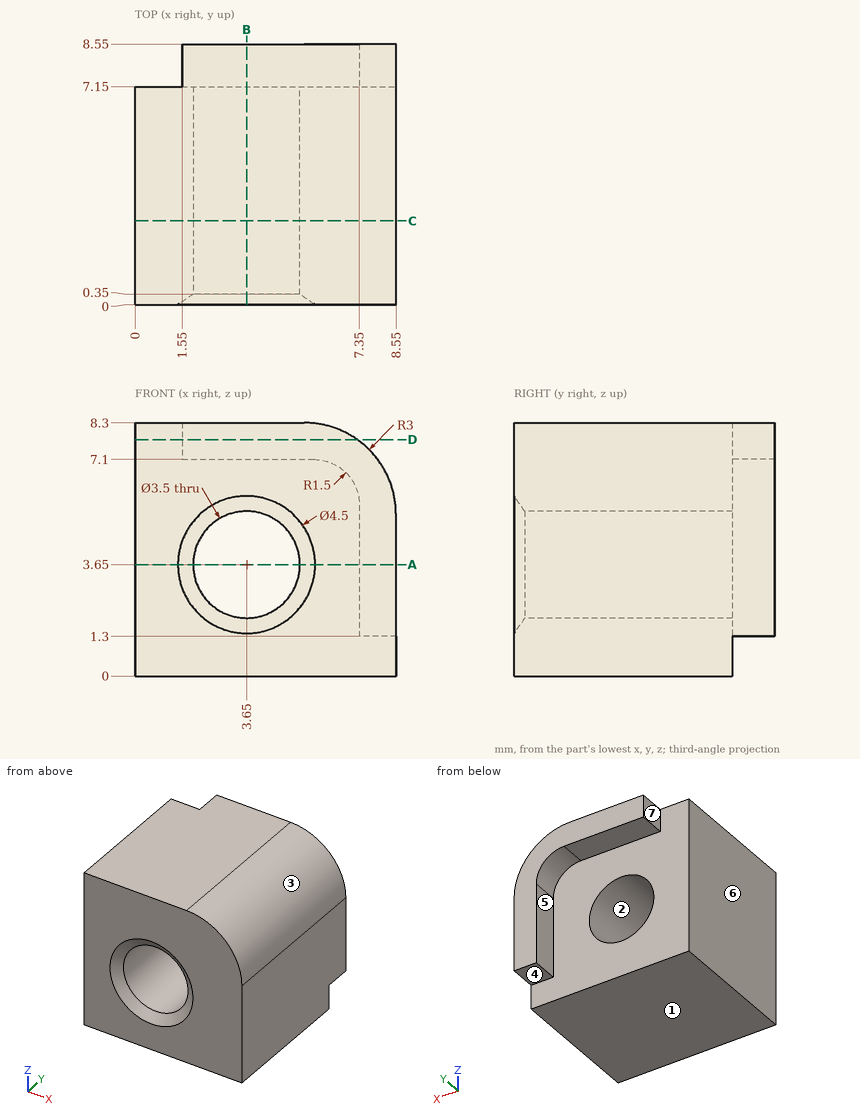
Input: dimensioned drawing with shaded views. Units: mm. Origin: part minimum x, y, z. A direction names the side the tool comes from. Give positions to 0.01 mm unless a question says otherwise; leave off trailing zeros. Order: outer loops, then holes, each group sorted by start corner. A loop starts at its lowest first (then second) coordinate and runs counter-clockwise, first axis right, second up. Notation, with made-up numbers: (68.25, -29.5) -> (85.25, -29.5) arc R20 cw to (85.25, -7.5) -> close; hole circle Ø3 at (-33, -33.5). An arc over 180 degrees is marked (long way). Use a Markdown table: item, result.
1) Ray query, line 1 along Z through (x, y) = (3.65, 3); line 2 along Y through (x, z) = (1, 0.5); line 3 along X through (y, z) = (1.5, 5.25). Return the intervals inside material, ascending. Write a range as [from, to].
Answer list:
| item | result |
|---|---|
| line 1 | [0, 1.9], [5.4, 8.3] |
| line 2 | [0, 7.15] |
| line 3 | [0, 2.94], [4.36, 8.55] |
2) Reachability of the marked faces 4, 5, 6 and 7 from +Z, -Z, +X, -X, +Y, -Y: full face, straight path, thin tool, end or side. Return the list, or none.
Answer list:
| item | result |
|---|---|
| face 4 | -Z, +X, -X, +Y |
| face 5 | -Z, -X, +Y |
| face 6 | +Z, -Z, -X, +Y, -Y |
| face 7 | +Z, -Z, -X, +Y |
3) Section query A-A, the plane z = 3.65. Return the cut outline in (x, y), then the cut area to 3 significant figures.
Answer list:
| item | result |
|---|---|
| outline | (0, 0) -> (1.4, 0) -> (1.9, 0.35) -> (1.9, 7.15) -> (0, 7.15) -> close; (5.4, 0.35) -> (5.9, 0) -> (8.55, 0) -> (8.55, 8.55) -> (7.35, 8.55) -> (7.35, 7.15) -> (5.4, 7.15) -> close |
| area | 37.6 mm² |
4) Contact query for flat-ended pins moving along their axis: P1, Ø1, axis at y = 4.5, z = 7, coming from the +X side; P2, Ø1, axis at y = 8, z = 7.5, coming from the -X side; P3, Ø1.5, axis at x = 4.5, z = 3.5, coming from the +Y side; P4, Ø1.5, axis at x = 3, y = 8, coming from the -Z side. Output: stop coordinate, or through.
Answer list:
| item | result |
|---|---|
| P1 | x = 8.3 |
| P2 | x = 1.55 |
| P3 | through |
| P4 | z = 7.1 |
5) Mould query, pull axis X, two halves, no side actions, for the marked faces 1, 2 and 3. Classes: +X half, -X half, draft (parallel to the pull), parting line (faces both ways), or undercut.
Answer list:
| item | result |
|---|---|
| face 1 | draft |
| face 2 | undercut |
| face 3 | +X half |
6) Section query C-C, the plane y = 2.75. Return the cut outline in (x, z), then the cut area to 3 significant figures.
Answer list:
| item | result |
|---|---|
| outline | (0, 0) -> (8.55, 0) -> (8.55, 5.3) arc R3 ccw to (5.55, 8.3) -> (0, 8.3) -> close; hole circle Ø3.5 at (3.65, 3.65) |
| area | 59.4 mm² |
7) Section query B-B, the plane x = 3.65. Return the cut outline in (y, z).
Answer list:
| item | result |
|---|---|
| outline | (0, 0) -> (7.15, 0) -> (7.15, 1.9) -> (0.35, 1.9) -> (0, 1.4) -> close; (0, 5.9) -> (0.35, 5.4) -> (7.15, 5.4) -> (7.15, 7.1) -> (8.55, 7.1) -> (8.55, 8.3) -> (0, 8.3) -> close |
8) Section query D-D, the plane z = 7.75. Return the cut outline in (x, y).
Answer list:
| item | result |
|---|---|
| outline | (0, 0) -> (7.28, 0) -> (7.28, 8.55) -> (1.55, 8.55) -> (1.55, 7.15) -> (0, 7.15) -> close |
